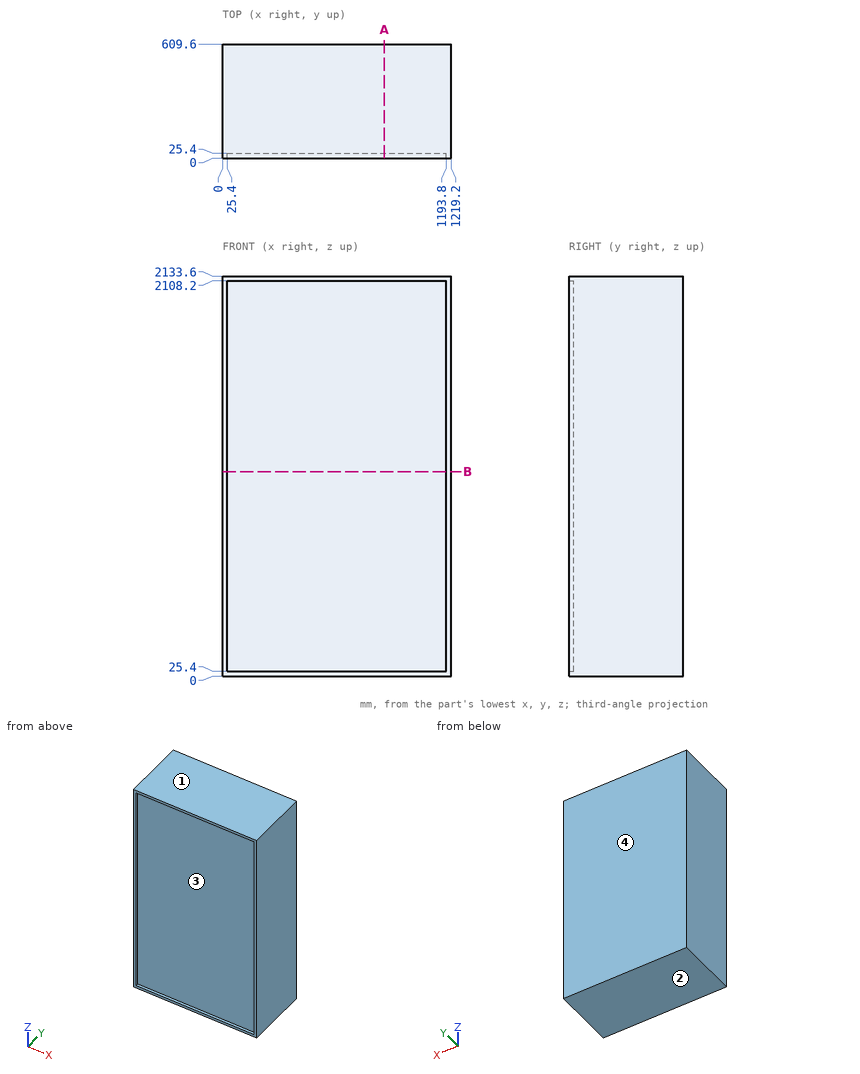
For this review, use the dimensioned drawing (mm, ordinates from the lowest corner) and the shaded views. Give positions to 0.01 mm unless a question says otherwise; leave off trailing zeros. Write each loop counter-clockwise with the first axis right and the second up, starting at its lowest first coordinate (ties: lowest second). Pieces come first, ordered by that corner, then holes.
(1) Consider section B-B, the plane z = 1091. Give the boundary of the cut face in (x, y).
(2) To check wall thickness, follow L1, parallel to Y at x = 579.5, z = 608.5. State the ranges of the line that lie inside material, in increasing order.
(3) The part is to be moulded in two halves that separate along Z. For the marked faces 1, 2, 3 and 4, say which applies: released by +Z, released by -Z, zero draft, split by the parting line, or undercut.
(4) For P1, Ø3, axis at x = 667.5, z = 729, coming from the -Y side, flat-tipped, find the tip position at first contact; note if it passes through.
(5) Consider section A-A, the plane x = 863. Give the boundary of the cut face in (y, z), and give its area (3 significant figures).
Returned:
1. outline: (0, 0) - (25.4, 0) - (25.4, 25.4) - (1193.8, 25.4) - (1193.8, 0) - (1219.2, 0) - (1219.2, 609.6) - (0, 609.6) - close
2. L1: y = 25.4 to 609.6
3. face 1: released by +Z
3. face 2: released by -Z
3. face 3: undercut
3. face 4: zero draft
4. P1: stops at y = 25.4
5. outline: (0, 0) - (609.6, 0) - (609.6, 2133.6) - (0, 2133.6) - (0, 2108.2) - (25.4, 2108.2) - (25.4, 25.4) - (0, 25.4) - close
5. area: 1,250,000 mm2
